Source: CAD feature listing. Evaluate the final solid. Frame: model axes, mm. Face numbers are marked on the shaded views. A direction names the side the tool comes from. Give positions to 0.01 mm unless a question says otherwise; leave off trailing zeros. Write each loop counter-clockwise with the first axis right and the second up, starting at its lowest first coordinate (ties: lowest second). Pieces come first, ordered by that corner, then holes. Notation, with made-up numbers: (-1, 68) -> (54, 68) arc R11 cw to (54, 74) -> close; hole circle Ø11 at (83.5, 81). An arc over 180 degrees is marked (long way). Use a Markdown table: item, result. Add a question column.
```python
from build123d import *

# Parameters (mm, degrees)
F1_DEPTH = 6.35
F2_R     = 6.3499
F0_R     = 5.08
F3_DEPTH = 6.35
F0_R_2   = 4.826
F4_DEPTH = 6.35
F5_DEPTH = 6.35


# Not quite as in the source:
# - a fillet or chamfer is up to 0.001 mm smaller than in the source, because OpenCascade refuses the exact size


with BuildPart() as f1:
    # F0 (on Front) → F1 (new body, symmetric)
    with BuildSketch(Plane.XZ):
        with BuildLine():
            Line((15.875, 6.35), (-15.875, 6.35))
            ThreePointArc((-15.875, 6.35), (-14.2195407024, 3.3649028089), (-13.646147458, 0))
            ThreePointArc((-13.646147458, 0), (-14.2195407024, -3.3649028089), (-15.875, -6.35))
            Line((-15.875, -6.35), (15.875, -6.35))
            ThreePointArc((15.875, -6.35), (13.646147458, 0), (15.875, 6.35))
        make_face()
    extrude(amount=F1_DEPTH, both=True)

    # F2 (radius 6.35 in the source; OpenCascade refuses exactly that, so slightly less here)
    f2_edges = [f1.edges().sort_by_distance(p)[0] for p in [
        (0, -6.35, 6.35),
        (0, 6.35, 6.35),
        (0, -6.35, -6.35),
        (0, 6.35, -6.35),
    ]]
    fillet(f2_edges, radius=F2_R)

    # F0 (on Front) → F3 (join)
    with BuildSketch(Plane.XZ):
        with BuildLine():
            ThreePointArc((33.966147458, 0), (27.1710502669, 9.5866067556), (15.875, 6.35))
            Line((15.875, 6.35), (15.875, -6.35))
            ThreePointArc((15.875, -6.35), (27.1710502669, -9.5866067556), (33.966147458, 0))
        make_face()
        with Locations((23.806147458, 0)):
            Circle(F0_R, mode=Mode.SUBTRACT)
        with BuildLine():
            Line((15.875, -6.35), (15.875, 6.35))
            ThreePointArc((15.875, 6.35), (13.646147458, 0), (15.875, -6.35))
        make_face()
    extrude(amount=F3_DEPTH)

    # F0 (on Front) → F4 (join)
    with BuildSketch(Plane.XZ):
        with BuildLine():
            Line((-15.875, -6.35), (-15.875, 6.35))
            ThreePointArc((-15.875, 6.35), (-33.966147458, 0), (-15.875, -6.35))
        make_face()
        with Locations((-23.806147458, 0)):
            Circle(F0_R_2, mode=Mode.SUBTRACT)
        with BuildLine():
            ThreePointArc((-13.646147458, 0), (-14.2195407024, 3.3649028089), (-15.875, 6.35))
            Line((-15.875, 6.35), (-15.875, -6.35))
            ThreePointArc((-15.875, -6.35), (-14.2195407024, -3.3649028089), (-13.646147458, 0))
        make_face()
    extrude(amount=-F4_DEPTH)

    # F0 (on Front) → F5 (join, symmetric)
    with BuildSketch(Plane.XZ):
        with Locations((-23.806147458, 0)):
            Circle(F0_R_2)
    extrude(amount=F5_DEPTH, both=True)


solid = f1.part
```
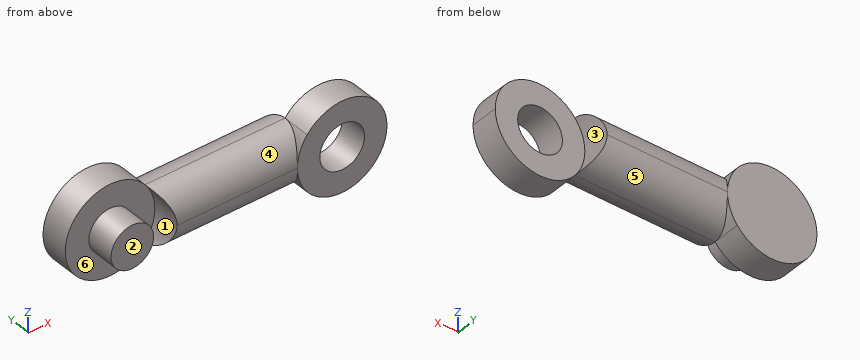
(1) First-contact query: pin 1 Ø5 at (x, y) = (20.5, 1.5) entering from +Z; pin 2 Ø6 at (y, z) = (5, -6.5) entering from +X; pin 3 Ø1 at (y, z) = (2.5, -8) entering from -X. Flat tips, straight axial feed; report the tip coordinate or a pass-through.
(2) Cut plane D-D on y = 4.5. Return the cut outline in (x, z) (3 decimals).
(3) Mould query, pull axis X, two halves, no side actions, for the marked faces 1, 2 and 3. Classes: +X half, -X half, draft (parallel to the pull), parting line (faces both ways), or undercut.
(4) Cut plane B-B on x = 24.5. Return the cut outline in (y, z).
(5) Access query for the marked faces 4, 5 and 6. Directions: +Z, -Z, +X, -X, +Y, -Y. A direction counts if a zero-diameter tool reaches every point of the face in a straight line with its end or side. Return the directions, or none.
(6) Cut plane A-A on z = -8.5. Return the cut outline in (x, y), then the cut area to 3 significant figures.
(7) Cut plane C-C on x = -24. Return the cut outline in (y, z).
(8) Material intervals for L1, parallel to X at y = -4.5, z = -0.75; L2, parallel to X at y = -1.75, z = 1.25; L3, parallel to Y at x = -24, z = -7, sorted ascending.
Output:
| question | item | result |
|---|---|---|
| 1 | pin 1 | z = 10.08 |
| 1 | pin 2 | x = 15.62 |
| 1 | pin 3 | x = -30.66 |
| 2 | outline | (-14.687, -4.48) -> (14.687, -4.48) arc R10.16 cw to (14.687, 4.48) -> (-14.687, 4.48) arc R10.16 ccw (long way) to start |
| 3 | face 1 | undercut |
| 3 | face 2 | draft |
| 3 | face 3 | +X half |
| 4 | outline | (-6.35, -10.14) -> (0, -10.14) -> (0, -5.03) -> (-6.35, -5.03) -> close; (-6.35, 5.03) -> (0, 5.03) -> (0, 10.14) -> (-6.35, 10.14) -> close |
| 5 | face 4 | +Z, -Y |
| 5 | face 5 | -Z, +X, +Y |
| 5 | face 6 | -Y |
| 6 | outline | (-29.37, 0) -> (-18.24, 0) -> (-18.24, 6.35) -> (-29.37, 6.35) -> close; (18.24, -6.35) -> (29.37, -6.35) -> (29.37, 0) -> (18.24, 0) -> close |
| 6 | area | 141 mm^2 |
| 7 | outline | (-6.35, -4.82) -> (0, -4.82) -> (0, -10.16) -> (6.35, -10.16) -> (6.35, 10.16) -> (0, 10.16) -> (0, 4.82) -> (-6.35, 4.82) -> close |
| 8 | L1 | -28.57 to -19.04, -13.67 to 18.78, 28.83 to 33.94 |
| 8 | L2 | -28.47 to -19.14, -13.72 to 18.88, 28.73 to 33.89 |
| 8 | L3 | 0 to 6.35 |
